```python
from build123d import *

# Parameters (mm, degrees)
F1_DEPTH = 152.4
F2_DEPTH = 139.7


with BuildPart() as f1:
    # F0 (on Top) → F1 (new body, symmetric)
    with BuildSketch(Plane.XY):
        with BuildLine():
            Line((-77.723362, 0), (11.176638, 0))
            Line((11.176638, 0), (11.176638, 242.86254))
            ThreePointArc((11.176638, 242.86254), (8.001638, 242.663321), (4.826638, 242.86254))
            Line((4.826638, 242.86254), (4.826638, 6.35))
            Line((4.826638, 6.35), (-71.373362, 6.35))
            Line((-71.373362, 6.35), (-71.373362, 146.409275))
            Line((-71.373362, 146.409275), (-77.723362, 146.409275))
            Line((-77.723362, 146.409275), (-77.723362, 0))
        make_face()
        with BuildLine():
            ThreePointArc((4.826638, 242.86254), (8.001638, 242.663321), (11.176638, 242.86254))
            Line((11.176638, 242.86254), (11.176638, 268.063321))
            Line((11.176638, 268.063321), (4.826638, 268.063321))
            Line((4.826638, 268.063321), (4.826638, 242.86254))
        make_face()
    extrude(amount=F1_DEPTH, both=True)

    # F0 (on Top) → F2 (join, symmetric)
    with BuildSketch(Plane.XY):
        with BuildLine():
            Line((11.176638, 268.063321), (11.176638, 242.86254))
            ThreePointArc((11.176638, 242.86254), (27.051638, 251.262801), (33.401638, 268.063321))
            ThreePointArc((33.401638, 268.063321), (-8.798883, 287.113321), (4.826638, 242.86254))
            Line((4.826638, 242.86254), (4.826638, 268.063321))
            Line((4.826638, 268.063321), (11.176638, 268.063321))
        make_face()
    extrude(amount=F2_DEPTH, both=True)


solid = f1.part
```
Read the model definition and answer for the solid it produces. Units are mm, in the model's axes. A direction names the side the tool comes from. Give positions to 0.01 mm unless a question says otherwise; leave off trailing zeros. Write each loop counter-clockwise with the first axis right and the second up, starting at its lowest first coordinate (ties: lowest second). Pieces come first, ordered by that corner, then holes. Notation, with made-up numbers: (22.5, -28.75) - (76.5, -28.75) arc R20 ccw to (76.5, -12.75) - close; hole circle Ø3 at (36.25, 30). An arc over 180 degrees is marked (long way). Write item = value, one per line. Start each with the question number.
Item 1: Find section A-A (y = 98). Give the vertices of the cut face in (x, z), then the cut area to 3 significant figures.
Item 2: Find section C-C (x = 0). Give the vertices of the cut face in (y, z), then the cut area to 3 significant figures.
Item 3: A tool of negligible diameter and unlimited length cuts with its end or side. For faces 1 (the flat face through (-33, 6.35, 2)), 2 (the flat face through (6, 85, 152.4)), from which of +Z, -Z, +X, -X, +Y, -Y can it reach the whole face along a straight path? Write none if from no direction.
Item 4: Find section D-D (y = 193). Give the vertices of the cut face in (x, z), then the cut area to 3 significant figures.
Item 5: The mould has two halves that part along X. Classify faces 3 (the flat face through (8, 269, 139.7)), 4 (the flat face through (-71.373, 75, 2)), 5 (the flat face through (4.827, 110, 2)), 6 (the flat face through (11.177, 132, 2)): +X half, -X half, draft (parallel to the pull), parting line (faces both ways), or undercut.
Item 6: Each of these flat-tipped pins is pushed along its axis until it touches: P1, Ø4, axis at x = 5, z = -9.5, coming from the +Y side; P2, Ø4, axis at x = -36, z = 15, coming from the +Y side; P3, Ø5, axis at x = 9.5, z = -147, coming from the +Y side. Where does it stop, or does it pass through?
Item 7: Find the intervals of material crossed by probe 1 along X at (y, z) = (97, -8); probe 2 along Y at (x, z) = (-31, 119); probe 3 along Y at (x, z) = (9, -118), in increasing order. Write a range as [from, to].
Item 8: Find section B-B (z = -27). Give the vertices of the cut face in (x, y), then the cut area to 3 significant figures.
Response:
q1.outline = (-77.72, -152.4) - (-71.37, -152.4) - (-71.37, 152.4) - (-77.72, 152.4) - close; (4.83, -152.4) - (11.18, -152.4) - (11.18, 152.4) - (4.83, 152.4) - close
q1.area = 3,870 mm²
q2.outline = (0, -152.4) - (6.35, -152.4) - (6.35, 152.4) - (0, 152.4) - close; (243.96, -139.7) - (292.17, -139.7) - (292.17, 139.7) - (243.96, 139.7) - close
q2.area = 15,400 mm²
q3.face_1 = +Z, -Z
q3.face_2 = +Z, +X, -X, +Y, -Y
q4.outline = (4.83, -152.4) - (11.18, -152.4) - (11.18, 152.4) - (4.83, 152.4) - close
q4.area = 1,940 mm²
q5.face_3 = draft
q5.face_4 = undercut
q5.face_5 = undercut
q5.face_6 = +X half
q6.P1 = 293.44
q6.P2 = 6.35
q6.P3 = 268.06
q7.probe_1 = [-77.72, -71.37], [4.83, 11.18]
q7.probe_2 = [0, 6.35]
q7.probe_3 = [0, 293.44]
q8.outline = (-77.72, 0) - (11.18, 0) - (11.18, 242.86) arc R25.4 ccw to (33.4, 268.06) arc R25.4 ccw (long way) to (4.83, 242.86) - (4.83, 6.35) - (-71.37, 6.35) - (-71.37, 146.41) - (-77.72, 146.41) - close
q8.area = 4,980 mm²
